```python
from build123d import *

# Parameters (mm, degrees)
BOSS_EXTRUDE1_DEPTH          = 12
SKETCH2_R                    = 10
BOSS_EXTRUDE2_DEPTH          = 8
F_5_0_5_DIAMETER_HOLE1_D     = 5
F_5_0_5_DIAMETER_HOLE1_DEPTH = 25
F_5_0_5_DIAMETER_HOLE1_TIP   = 1.502151548
SKETCH6_R                    = 1.5
CUT_EXTRUDE1_DEPTH           = 11
SKETCH8_R                    = 1.5
CUT_EXTRUDE2_DEPTH           = 4


with BuildPart() as part:
    # Sketch1 → Boss-Extrude1 (new body)
    with BuildSketch(Plane.XY.offset(26)):
        with BuildLine():
            Line((4.873707659, 0), (6.190281068, 0.43286662))
            ThreePointArc((6.190281068, 0.43286662), (6.091386481, 1.184045587), (5.901683351, 1.917573162))
            Line((5.901683351, 1.917573162), (4.502718754, 1.865087175))
            ThreePointArc((4.502718754, 1.865087175), (4.052339818, 2.7076869), (3.446231735, 3.446231735))
            Line((3.446231735, 3.446231735), (4.071106798, 4.683272643))
            ThreePointArc((4.071106798, 4.683272643), (3.470014023, 5.144507351), (2.817191332, 5.529049304))
            Line((2.817191332, 5.529049304), (1.865087175, 4.502718754))
            ThreePointArc((1.865087175, 4.502718754), (0.950813197, 4.780060733), (0, 4.873707659))
            Line((0, 4.873707659), (-0.43286662, 6.190281068))
            ThreePointArc((-0.43286662, 6.190281068), (-1.184045587, 6.091386481), (-1.917573162, 5.901683351))
            Line((-1.917573162, 5.901683351), (-1.865087175, 4.502718754))
            ThreePointArc((-1.865087175, 4.502718754), (-2.7076869, 4.052339818), (-3.446231735, 3.446231735))
            Line((-3.446231735, 3.446231735), (-4.683272643, 4.071106798))
            ThreePointArc((-4.683272643, 4.071106798), (-5.144507351, 3.470014023), (-5.529049304, 2.817191332))
            Line((-5.529049304, 2.817191332), (-4.502718754, 1.865087175))
            ThreePointArc((-4.502718754, 1.865087175), (-4.780060733, 0.950813197), (-4.873707659, 0))
            Line((-4.873707659, 0), (-6.190281068, -0.43286662))
            ThreePointArc((-6.190281068, -0.43286662), (-6.091386481, -1.184045587), (-5.901683351, -1.917573162))
            Line((-5.901683351, -1.917573162), (-4.502718754, -1.865087175))
            ThreePointArc((-4.502718754, -1.865087175), (-4.052339818, -2.7076869), (-3.446231735, -3.446231735))
            Line((-3.446231735, -3.446231735), (-4.071106798, -4.683272643))
            ThreePointArc((-4.071106798, -4.683272643), (-3.470014023, -5.144507351), (-2.817191332, -5.529049304))
            Line((-2.817191332, -5.529049304), (-1.865087175, -4.502718754))
            ThreePointArc((-1.865087175, -4.502718754), (-0.950813197, -4.780060733), (0, -4.873707659))
            Line((0, -4.873707659), (0.43286662, -6.190281068))
            ThreePointArc((0.43286662, -6.190281068), (1.184045587, -6.091386481), (1.917573162, -5.901683351))
            Line((1.917573162, -5.901683351), (1.865087175, -4.502718754))
            ThreePointArc((1.865087175, -4.502718754), (2.7076869, -4.052339818), (3.446231735, -3.446231735))
            Line((3.446231735, -3.446231735), (4.683272643, -4.071106798))
            ThreePointArc((4.683272643, -4.071106798), (5.144507351, -3.470014023), (5.529049304, -2.817191332))
            Line((5.529049304, -2.817191332), (4.502718754, -1.865087175))
            ThreePointArc((4.502718754, -1.865087175), (4.780060733, -0.950813197), (4.873707659, 0))
        make_face()
    extrude(amount=-BOSS_EXTRUDE1_DEPTH)

    # Sketch2 → Boss-Extrude2 (add)
    with BuildSketch(Plane.XY.offset(26)):
        Circle(SKETCH2_R)
    extrude(amount=BOSS_EXTRUDE2_DEPTH)

    # Ø5.0 (5) Diameter Hole1
    with Locations(Plane(origin=(0, 0, 14), x_dir=(-1, 0, 0), z_dir=(0, 0, -1))):
        with Locations((0, 0)):
            Hole(F_5_0_5_DIAMETER_HOLE1_D / 2, depth=F_5_0_5_DIAMETER_HOLE1_DEPTH)
            with Locations((0, 0, -(F_5_0_5_DIAMETER_HOLE1_DEPTH + F_5_0_5_DIAMETER_HOLE1_TIP / 2))):  # 118° drill point
                Cone(0, F_5_0_5_DIAMETER_HOLE1_D / 2, F_5_0_5_DIAMETER_HOLE1_TIP, mode=Mode.SUBTRACT)

    # Sketch6 → Cut-Extrude1 (cut)
    with BuildSketch(Plane(origin=(0, 0, 0), x_dir=(1, 0, 0), z_dir=(0, 1, 0))):
        with Locations(Location((0, -30.5, 0), (0, 0, 90))):
            Circle(SKETCH6_R)
    extrude(amount=CUT_EXTRUDE1_DEPTH, mode=Mode.SUBTRACT)

    # Sketch8 → Cut-Extrude2 (cut)
    with BuildSketch(Plane(origin=(0, 3.5, 0), x_dir=(-1, 0, 0), z_dir=(0, 1, 0))):
        Polygon((-2.75, 32.08771324), (-2.75, 34), (2.75, 34), (2.75, 32.08771324), (2.75, 28.91228676), (0, 27.324573519), (-2.75, 28.91228676), align=None)
        with Locations(Location((0, 30.5, 0), (0, 0, 270))):
            Circle(SKETCH8_R, mode=Mode.SUBTRACT)
    extrude(amount=CUT_EXTRUDE2_DEPTH, mode=Mode.SUBTRACT)


solid = part.part
```
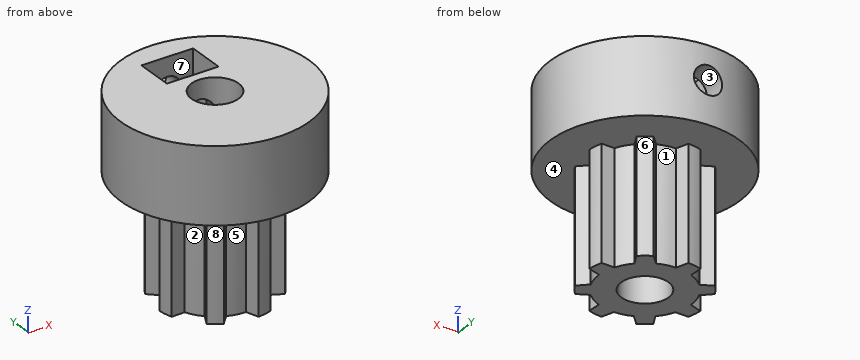
Read the model definition and answer for the solid it produces. Units are mm, in the model's axes. Face numbers are marked on the shaded views. A direction names the side the tool comes from. Round coordinates to 2 decimals unless told otherwise and drop trailing zeros. Write each loop counter-clockwise with the first axis right and the second up, starting at its lowest first coordinate (ties: lowest second). Pieces come first, ordered by that corner, then holes. Notation, with made-up numbers: M -1,10.5 L 30,10.5 A36 ccw 30,44.5 Z; hole C -10.5,78 d1. An arc over 180 degrees is marked long. One line per item, written item: value.
Q1. Which of the six approach directions +Z, -Z, +X, -X, +Y, -Y give full straight-line access (tool end or side, diameter ignored) to the marked faces 4, 5, 6, 7 and 8?
Data:
face 4: -Z
face 5: -Z, -Y
face 6: -Z, +X, +Y
face 7: +Z
face 8: -Z, -X, -Y
Q2. For a pull along Y with two mould halves and no side action, classify the marked faces 1, 2 and 3 as +Y half, -Y half, draft (parallel to the pull), parting line (faces both ways), or undercut.
Data:
face 1: +Y half
face 2: undercut
face 3: draft
Q3. Flat-ended cylindrical pins translate along their axes: pin 1 Ø1.5 at (x, y) = (8, 2) entering from -Z; pin 2 Ø6 at (x, z) = (1.5, 17.5) entering from +Y; pin 3 Ø4.5 at (y, z) = (5, 30.5) entering from +X. Find the tip coordinate at first contact, or state that the pin passes through.
Data:
pin 1: z = 26
pin 2: y = 6.19
pin 3: x = 9.61
Q4. Straight lines are drawn through the part: line 1 (X direction, y = 3.5, z = 16.75); line 2 (Z direction, x = 8, y = 0.5); line 3 (X direction, y = 1.75, z = 28). For each, find the intervals that lie inside material, in ascending order. Write a range as [from, to].
Data:
line 1: [-5.12, -3.55], [-3.39, 3.47]
line 2: [26, 34]
line 3: [-9.85, -1.79], [1.79, 9.85]
Q5. Find section C-C on y = -5.25. Write down the section's boundary in (x, z).
Data:
outline: M -8.51,26 L -3.31,26 L -3.31,14 L -2.56,14 L -2.56,26 L 0.12,26 L 0.12,14 L 1.89,14 L 1.89,26 L 8.51,26 L 8.51,34 L -8.51,34 Z
Q6. Find section D-D on x = -6.75. Write down the section's boundary in (y, z), plus the area to 3 significant figures.
Data:
outline: M -7.38,26 L 7.38,26 L 7.38,34 L -7.38,34 Z
area: 118 mm2
Q7. Find section B-B on z = 28.5. Write down the section's boundary in (x, y).
Data:
outline: C 0,0 d20; hole C 0,0 d5; hole M -2.04,3.5 L 2.04,3.5 L 2.04,7.5 L -2.04,7.5 Z
